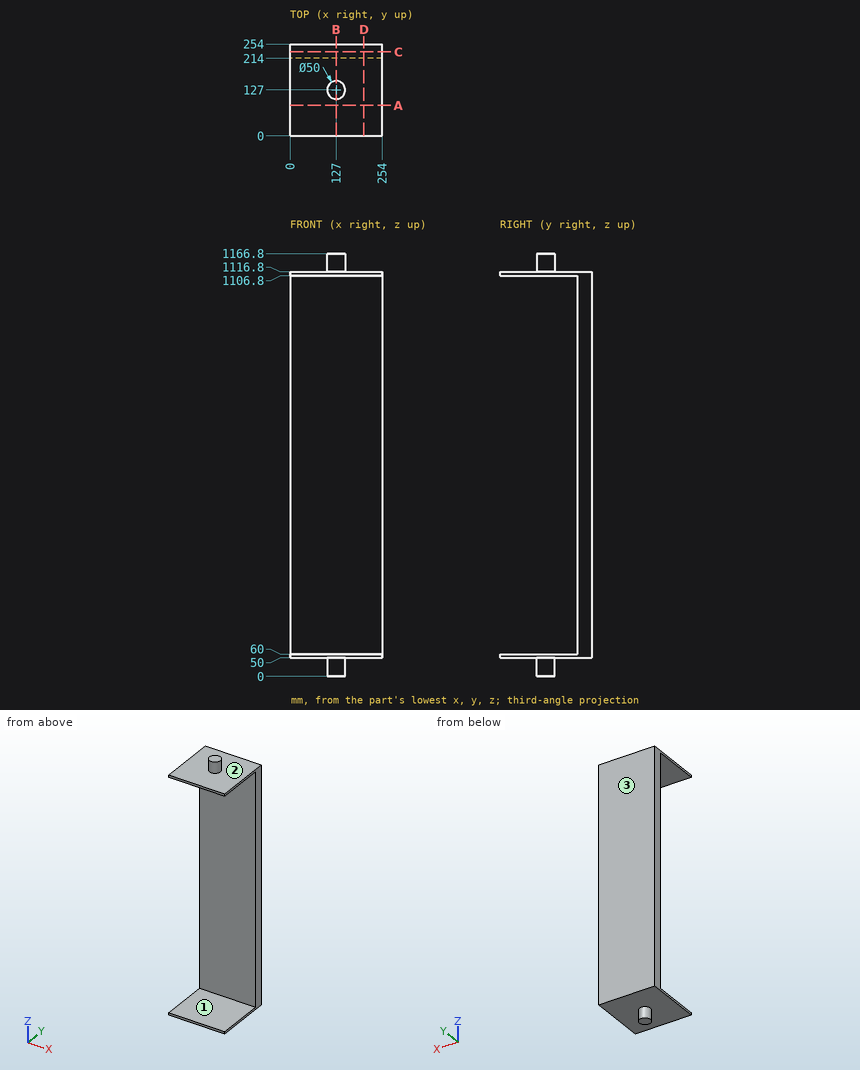
The figure shows three views and two pictorial views of one solid part (mm, origin at its lowest corner). Answer the questions. Round coordinates to 2 decimals unless told otherwise and drop trailing zeros. Write each loop counter-clockwise with the first axis right and the second up, starting at its lowest first coordinate (ties: lowest second). Pieces come first, ordered by that corner, then holes. Notation, with made-up numbers: (78, 28) -> (135, 28) arc R20 cw to (135, 42) -> close; hole circle Ø3 at (40.25, 64). An arc over 180 degrees is marked (long way). Answer as a JSON object with one key per item and string values. Group by question number.
Q1. Section D-D (x = 204) is taken. Write down the section's boundary in (y, z).
Q2. Straight lines are drawn through the part: line 1 along Z through (x, y) = (43, 66.5); line 2 along Y through (x, z) = (120, 780); line 3 along Z through (x, y) = (111.5, 128). For each, find the intervals that lie inside material, in ascending order.
Q3. Section B-B (x = 127) is taken. Write down the section's boundary in (y, z), plus the area to 3 significant figures.
Q4. Section C-C (y = 232) is taken. Write down the section's boundary in (x, z).
Q5. Determine the mould class of the marked faces 1, 2 and 3 for opening direction Z: pulls with the +Z half, pulls with the -Z half, needs draft (parallel to the pull), parting line crosses it, or undercut.
Q6. Section A-A (y = 84.5) is taken. Write down the section's boundary in (x, z).
Q7. Each of these flat-tipped pins is pushed along its axis until it touches: pin 1 Ø10 at (x, y) = (147, 79) entering from +Z; pin 2 Ø1.5 at (x, y) = (176, 39.5) entering from -Z. Where does it stop, or does it pass through?
Check values:
{
 "1": {"outline": "(0, 50) -> (254, 50) -> (254, 1116.8) -> (0, 1116.8) -> (0, 1106.8) -> (214, 1106.8) -> (214, 60) -> (0, 60) -> close"},
 "2": {"line 1": "50 to 60, 1106.8 to 1116.8", "line 2": "214 to 254", "line 3": "0 to 60, 1106.8 to 1166.8"},
 "3": {"outline": "(0, 50) -> (102, 50) -> (102, 0) -> (152, 0) -> (152, 50) -> (254, 50) -> (254, 1116.8) -> (152, 1116.8) -> (152, 1166.8) -> (102, 1166.8) -> (102, 1116.8) -> (0, 1116.8) -> (0, 1106.8) -> (214, 1106.8) -> (214, 60) -> (0, 60) -> close", "area": "52,000 mm^2"},
 "4": {"outline": "(0, 50) -> (254, 50) -> (254, 1116.8) -> (0, 1116.8) -> close"},
 "5": {"face 1": "undercut", "face 2": "pulls with the +Z half", "face 3": "needs draft"},
 "6": {"outline": "(0, 50) -> (254, 50) -> (254, 60) -> (0, 60) -> close; (0, 1106.8) -> (254, 1106.8) -> (254, 1116.8) -> (0, 1116.8) -> close"},
 "7": {"pin 1": "z = 1116.8", "pin 2": "z = 50"}
}
